from build123d import *

# Parameters (mm, degrees)
F1_DEPTH = 660.4
F3_DEPTH = 38.101
F4_R     = 4.7625
F5_DEPTH = 38.101


with BuildPart() as f1:
    # F0 (on Top) → F1 (new body)
    with BuildSketch(Plane.XY):
        Polygon((0, 3.175), (0, 0), (38.1, 0), (38.1, 38.1), (34.925, 38.1), (34.925, 3.175), align=None)
    extrude(amount=F1_DEPTH)

    # F2 (on face) → F3 (cut, through all)
    with BuildSketch(Plane.XZ):
        Polygon((0, 622.3), (38.1, 660.4), (0, 660.4), align=None)
        Polygon((0, 0), (38.1, 0), (0, 38.1), align=None)
    extrude(amount=-F3_DEPTH, mode=Mode.SUBTRACT)

    # F4 (on face) → F5 (cut, through all)
    with BuildSketch(Plane.XZ):
        with Locations((19.05, 45.990768)):
            Circle(F4_R)
        with Locations((19.05, 614.409232)):
            Circle(F4_R)
    extrude(amount=-F5_DEPTH, mode=Mode.SUBTRACT)


solid = f1.part
Geometry check sheet. Reference: the model listing, model coordinates, mm. A direction names the side the tool comes from. Coordinates: 2 decimals unless noted, no trailing zeros. Order: outer loops, then holes, each group sorted by start corner. A loop starts at its lowest first (then second) coordinate and runs counter-clockwise, first axis right, second up. Notation, with made-up numbers: (-23.75, 44.5) - (-3.75, 44.5) arc R4 ccw to (-3.75, 50.5) - close; hole circle Ø7 at (-4.75, -5.75). An arc over 180 degrees is marked (long way). One line per item, written item: value.
(1) Access from +Z, -Z, +X, -X, +Y, -Y to the whole of each face (thin tool, end or side, straight path). Record for faces 1 (the face through (27.6, 2, 10.5)), 2 (the face through (34.925, 21, 326)).
Data:
face 1: -Z, -X, +Y, -Y
face 2: +Z, -Z, -X, +Y
(2) Sectioned sample at B-B (y = 31). Enter the section's corners in (x, z) (3 decimals).
Data:
outline: (34.925, 3.175) - (38.1, 0) - (38.1, 660.4) - (34.925, 657.225) - close
(3) Thickness scan on probe 1 along Z at (x, y) = (19, 1); probe 2 along Z at (x, y) = (19.05, 0.7); probe 3 along Y at (x, z) = (22.5, 256) (3 decimals). Record the ranges inside material, lowest first. Write a range as from..to.
Data:
probe 1: z = 19.1..41.23, 50.75..609.65, 619.17..641.3
probe 2: z = 19.05..41.23, 50.75..609.65, 619.17..641.35
probe 3: y = 0..3.175
(4) Sectioned sample at A-A (z = 456). Enter the section's corners in (x, y) (3 decimals), and give its area (3 significant figures).
Data:
outline: (0, 0) - (38.1, 0) - (38.1, 38.1) - (34.925, 38.1) - (34.925, 3.175) - (0, 3.175) - close
area: 232 mm^2
(5) Depth check by flat-ended pin: pin 1 Ø1 at (y, z) = (24, 401) entering from -X (3 decimals); pin 2 Ø1 at (x, z) = (24.5, 182) entering from +Y (3 decimals). Enter the tip coordinate at first touch or a pass-through.
Data:
pin 1: stops at x = 34.925
pin 2: stops at y = 3.175
